The drawing under review shows one solid part. Ordinate dimensions are in mm from its lowest x, y, z. A direction names the side the tool comes from. Coordinates: 2 decimals unless noted, no trailing zeros. Order: outer loops, then holes, each group sorted by start corner. A loop starts at its lowest first (then second) coordinate and runs counter-clockwise, first axis right, second up.
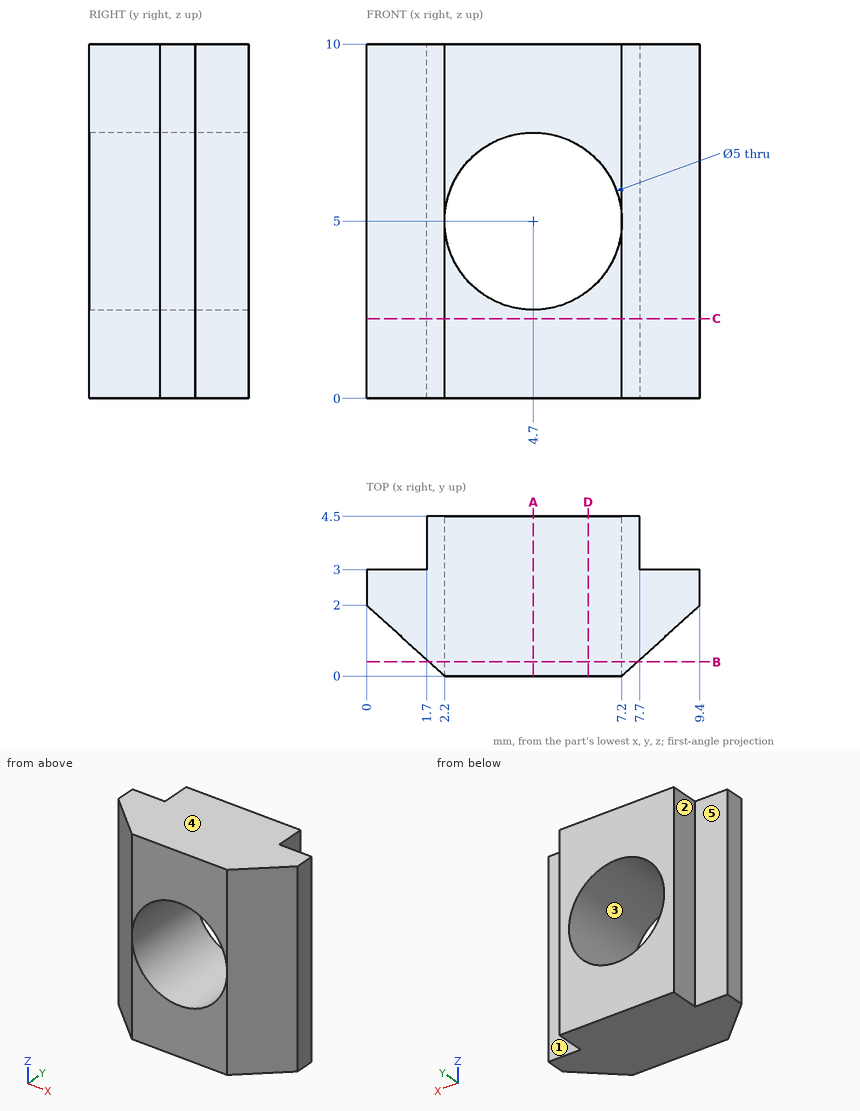
1. Add section B-B (y = 0.4). Give the boundary of the cut face in (x, z).
2. Mouldability with a two-part tool opening along X and no side actions: class the marked faces 1, 2 and 3 as pulls with the +X half, pulls with the -X half, needs draft (parallel to the pull), parting line crosses it, or undercut.
3. Add section A-A (x = 4.7). Give the boundary of the cut face in (y, z).
4. Add section D-D (x = 6.25). Give the boundary of the cut face in (y, z), and give its area (3 significant figures).
5. Add section C-C (z = 2.25). Give the boundary of the cut face in (x, y), and give its area (3 significant figures).
6. To check wall thickness, follow line 1 (Z direction, x = 4.7, y = 2.95); line 2 (X direction, y = 3.7, z = 1); line 3 (Z direction, x = 3.5, y = 1.4). State the ranges of each line that lie inside material, in increasing order.
7. For the marked faces 4 and 5, list the 3-axis set-ups (+Z, -Z, +X, -X, +Y, -Y) from which the entire face can be reached by the end or side of a thin tool; tool diameter is ignored.
8. Insertion check: pin 1 (1.9 mm diameter, centred on x = 9, z = 7.5, fed in from +Y); pin 2 (1.2 mm diameter, centred on y = 4, z = 6.5, fed in from -X). Each pin has a flat end and moves straight along its axis. Give the tip position at first contact, or say it passes through.
Solution:
1. outline: (1.76, 0) - (7.64, 0) - (7.64, 10) - (1.76, 10) - close; hole circle Ø5 at (4.7, 5)
2. face 1: needs draft
2. face 2: pulls with the -X half
2. face 3: undercut
3. outline: (0, 0) - (4.5, 0) - (4.5, 2.5) - (0, 2.5) - close; (0, 7.5) - (4.5, 7.5) - (4.5, 10) - (0, 10) - close
4. outline: (0, 0) - (4.5, 0) - (4.5, 3.04) - (0, 3.04) - close; (0, 6.96) - (4.5, 6.96) - (4.5, 10) - (0, 10) - close
4. area: 27.3 mm2
5. outline: (0, 2) - (2.2, 0) - (7.2, 0) - (9.4, 2) - (9.4, 3) - (7.7, 3) - (7.7, 4.5) - (1.7, 4.5) - (1.7, 3) - (0, 3) - close
5. area: 32.8 mm2
6. line 1: z = 0 to 2.5, 7.5 to 10
6. line 2: x = 1.7 to 7.7
6. line 3: z = 0 to 2.81, 7.19 to 10
7. face 4: +Z, +X, -X, +Y, -Y
7. face 5: +Z, -Z, -X, +Y
8. pin 1: stops at y = 3
8. pin 2: stops at x = 1.7
